Check sheet for the modelled part. Datum: model origin and axes. Units: mm. A direction names the side the tool comes from. Round coordinates to 2 decimals unless told otherwise and drop trailing zeros. Write each loop counter-clockwise with the first axis right and the second up, starting at its lowest first coordinate (ties: lowest second). Pieces come first, ordered by that corner, then holes.
Item 1: Material ranges on line 1 along X through (y, z) = (-38.5, 21.5); line 2 along Z through (x, y) = (42, -14.5), recorded low to high.
Item 2: Section check C-C, the plane x = 160.5. Record the cut outline in (y, z).
Item 3: Section check B-B, the plane y = -17. Record the cut outline in (x, z) (3 decimals).
Item 4: Set-up check for faces 4 (the flat face through (304.8, -25, 22)), 5 (the flat face through (2.21, -25, 23)): record each of +Z, -Z, +X, -X, +Y, -Y from which the full face is reachable in a straight line by a thin tool's end or side.
Item 5: Section check A-A, the plane z = 19. Record the cut outline in (x, y), plus the area to 3 significant figures.
Item 6: Depth check by flat-ended pin: pin 1 (5 mm diameter, centred on x = 221, y = -33, fed in from +Z). Enter the tip coordinate at first touch or a pass-through.
Item 7: Release check for a two-part mould opening along X. For faces 1 (the flat face through (0, -26, 22)), 2 (the flat face through (153, -50.8, 1)), 3 (the flat face through (302.59, -25, 23)) record: pulls with the +X half, pulls with the -X half, needs draft (parallel to the pull), parting line crosses it, or undercut.
Autodesk Inventor part; units mm, degrees
ref_plane "YZ Plane" through (0, 0, 0) normal (1, 0, 0) x (0, 1, 0)
ref_plane "XZ Plane" through (0, 0, 0) normal (0, 1, 0) x (-1, 0, 0)
ref_plane "XY Plane" through (0, 0, 0) normal (0, 0, 1) x (1, 0, 0)
sketch "Sketch1" plane through (0, 0, 0) normal (0, 0, 1) x (1, 0, 0)
  line L0 (0, 0) -> (304.8, 0)
  line L1 (304.8, 0) -> (304.8, -50.8)
  line L2 (304.8, -50.8) -> (0, -50.8)
  line L3 (0, -50.8) -> (0, 0)
  dimension "d0" = 304.8
  dimension "d1" = 50.8
extrude "Extrusion1" add sketch "Sketch1" along normal blind 2.2098
sketch "Sketch2" plane through (0, 0, 2.2098) normal (0, 0, 1) x (1, 0, 0)
  line L0 (0, -50.8) -> (304.8, -50.8)
  line L1 (0, 0) -> (2.2098, 0)
  line L2 (2.2098, 0) -> (2.2098, -50.8)
  line L3 (2.2098, -50.8) -> (0, -50.8)
  line L4 (0, -50.8) -> (0, 0)
  line L5 (304.8, 0) -> (302.5902, 0)
  line L6 (302.5902, 0) -> (302.5902, -50.8)
  line L7 (302.5902, -50.8) -> (304.8, -50.8)
  line L8 (304.8, -50.8) -> (304.8, 0)
  dimension "d4" = 2.2098
  dimension "d5" = 2.2098
extrude "Extrusion2" add sketch "Sketch2" along normal blind 50.8
fillet "Fillet1" radius 3.175 1 edges at (304.8, -25.4, 0)
fillet "Fillet2" radius 3.175 1 edges at (0, -25.4, 0)
fillet "Fillet3" radius 3.175 1 edges at (2.2098, -25.4, 2.2098)
fillet "Fillet4" radius 3.175 1 edges at (302.5902, -25.4, 2.2098)
sketch "Sketch3" plane through (304.8, -50.8, 53.0098) normal (1, 0, 0) x (0, 0, -1)
  line L0 (0, 0) -> (12.3698, 0)
  line L1 (49.8348, 0) -> (0, 0)
  line L2 (12.3698, 0) -> (12.3698, 65.8948)
  line L3 (47.625, 50.8) -> (0, 50.8)
  line L4 (12.3698, 65.8948) -> (-20.1931, 65.8948)
  line L5 (-20.1931, 65.8948) -> (-20.1931, 0)
  line L6 (-20.1931, 0) -> (12.3698, 0)
  point P0 (53.0098, 50.8)
  dimension "d12" = 12.3698
extrude "Extrusion3" cut sketch "Sketch3" against normal through all
properties part number "Conveyor Brace"
Values found:
1. line 1: x = 0 to 2.21, 302.59 to 304.8
1. line 2: z = 0 to 2.21
2. outline: (-50.8, 0) - (0, 0) - (0, 2.21) - (-50.8, 2.21) - close
3. outline: (0, 3.175) arc R3.175 ccw to (3.175, 0) - (301.625, 0) arc R3.175 ccw to (304.8, 3.175) - (304.8, 40.64) - (302.59, 40.64) - (302.59, 5.385) arc R3.175 cw to (299.415, 2.21) - (5.385, 2.21) arc R3.175 cw to (2.21, 5.385) - (2.21, 40.64) - (0, 40.64) - close
4. face 4: +Z, -Z, +X, +Y, -Y
4. face 5: +Z, +Y, -Y
5. outline: (0, -50.8) - (2.21, -50.8) - (2.21, 0) - (0, 0) - close; (302.59, -50.8) - (304.8, -50.8) - (304.8, 0) - (302.59, 0) - close
5. area: 225 mm2
6. pin 1: stops at z = 2.21
7. face 1: pulls with the -X half
7. face 2: needs draft
7. face 3: undercut
